```python
from build123d import *

# Parameters (mm, degrees)
BOSS_EXTRUDE2_DEPTH = 3.175
SKETCH6_W           = 3.175
SKETCH6_H           = 6.35
SKETCH6_W_2         = 12.7
SKETCH6_H_2         = 3.175
BOSS_EXTRUDE4_DEPTH = 3.175


with BuildPart() as part:
    # Sketch5 → Boss-Extrude2 (new body)
    with BuildSketch(Plane(origin=(0, 0, 0), x_dir=(1, 0, 0), z_dir=(0, 1, 0))):
        with BuildLine():
            Line((0, 0), (0, 19.05))
            add(Edge.make_bspline(
                [(34.925, 0), (34.925, 19.05), (0, 19.05)],
                knots=[3.141592654, 3.141592654, 3.141592654, 4.71238898, 4.71238898, 4.71238898], degree=2, weights=[1, 0.707106781, 1]))
            Line((34.925, 0), (0, 0))
        make_face()
    extrude(amount=BOSS_EXTRUDE2_DEPTH)

    # Sketch6 → Boss-Extrude4 (add)
    with BuildSketch(Plane(origin=(0, 3.175, 0), x_dir=(1, 0, 0), z_dir=(0, 1, 0))):
        with Locations((-1.5875, 8.255)):
            Rectangle(SKETCH6_W, SKETCH6_H)
        with Locations((16.51, -1.5875)):
            Rectangle(SKETCH6_W_2, SKETCH6_H_2)
    extrude(amount=-BOSS_EXTRUDE4_DEPTH)


solid = part.part
```
Input: part model. Units: mm. Frame: model coordinates. A direction names the side the tool comes from. Coordinates: 2 decimals unless noted, no trailing zeros. Loops run counter-clockwise (first coordinate to the right, second up) from the corner with the lowest first, then second, coordinate; pieces in that order, holes last. Notation, with made-up numbers: (69, 0.5) - (104, 0.5) arc R21 cw to (104, 33.5) - close; hole circle Ø9 at (-28, 84). An arc over 180 degrees is marked (long way). Answer in a Markdown table with one row per item.
(1) Cut plane A-A on z = 1.25. Output: boundary loops of the cut face in (x, y) (3 decimals).
Model answer:
| item | result |
|---|---|
| outline | (10.16, 0) - (22.86, 0) - (22.86, 3.175) - (10.16, 3.175) - close |
(2) Material intervals for L1, parallel to X at y = 1.85, z = 0.5; L2, parallel to Z at x = 16, y = 0.3 (3 decimals); L3, parallel to X at y = 1.55, z = -15, sorted ascending. Write a range as from..to.
Model answer:
| item | result |
|---|---|
| L1 | x = 10.16..22.86 |
| L2 | z = -16.933..3.175 |
| L3 | x = 0..21.53 |
(3) Set-up query: faces 1 (the face through (16, 3.175, -8)), 2 (the face through (-2, 2, -5.08)), 3 (the face through (0, 2, -15)), 4 (the face through (16, 2, 3.175)), 5 (the face through (22.86, 2, 2)). Return all of +Z, -Z, +X, -X, +Y, -Y with unobstructed straight access to the full face (end or side cutting, diameter ignored); none if empty.
Model answer:
| item | result |
|---|---|
| face 1 | +Z, -Z, +X, -X, +Y |
| face 2 | +Z, -X, +Y, -Y |
| face 3 | -Z, -X, +Y, -Y |
| face 4 | +Z, +X, -X, +Y, -Y |
| face 5 | +Z, +X, +Y, -Y |
(4) Pin query (flat end, axial travel): P1, Ø1, axis at y = 1.5, z = 1.5, coming from the -X side; P2, Ø1, axis at x = 30, y = 2, coming from the +Z side; P3, Ø1, axis at y = 1.5, z = -2.5, coming from the -X side. Return the tip coordinate at first contact, or that it passes through.
Model answer:
| item | result |
|---|---|
| P1 | stops at x = 10.16 |
| P2 | stops at z = 0 |
| P3 | stops at x = 0 |
